Source: CAD feature listing. Evaluate the final solid. Frame: model axes, mm. A direction names the side the tool comes from. Coordinates: 2 decimals unless noted, no trailing zeros. Write each loop counter-clockwise with the first axis right and the second up, starting at its lowest first coordinate (ties: lowest second). Pieces come first, ordered by that corner, then holes. Notation, with made-up numbers: M 57.25,2 L 106.25,2 A21 cw 106.25,12 Z; hole C 86,73 d2. An arc over 180 degrees is marked long. Answer as CSV lines item,"result". Start each with the question number.
1. Section C-C on z = -18. Return the cut outline in (x, y) (3 decimals).
2. Reachability of faces 4 (the face through (-47, 6.35, 0)), 5 (the face through (-7.7, 4.7, -10.1)) from +Z, -Z, +X, -X, +Y, -Y: full face, straight path, thin tool, end or side. Return the list, or none.
3. Section B-B on x = -9.5. Return the cut outline in (y, z) (3 decimals), plus the area to 3 significant figures.
4. Mould query, pull axis Z, two halves, no side actions, for faces 1 (the face through (-63.85, 1.57, -14.18)), 2 (the face through (0.109, 3.47, -3.046)), 3 (the face through (0, 6.35, 47)). Classes: pulls with the +Z half, pulls with the -Z half, needs draft (parallel to the pull), parting line crosses it, or undercut.
5. Section A-A on y = 2. Return the cut outline in (x, z) (3 decimals).
6. Line query: probe 1 along X at (y, z) = (3.55, 0); probe 2 along Y at (x, z) = (-44, -34) (3 decimals); probe 3 along X at (y, z) = (2.75, 1). Output: solid intervals per line, ascending. Write a range as [from, to].
7. Contact query for flat-ended pins moving along their axis: pin 1 Ø3.5 at (x, z) = (0, 0) entering from +Y; pin 2 Ø1.5 at (y, z) = (1.5, 8.5) entering from +X; pin 3 Ø12 at (x, z) = (-26, 24) entering from +Y (3 decimals); pin 4 Ø3 at (y, z) = (5, 29) entering from -X. Output: stop coordinate, or through.
8. Section D-D on x = 15. Return the cut outline in (y, z) (3 decimals), plus the area to 3 significant figures.
```python
from build123d import *

# Parameters (mm, degrees)
SKETCH1_R           = 65.405
BOSS_EXTRUDE1_DEPTH = 3.175
SKETCH2_R           = 12.7
BOSS_EXTRUDE2_DEPTH = 3.175
CUT_EXTRUDE1_DEPTH  = 5.842
SKETCH4_R           = 7.032250482
BOSS_EXTRUDE3_DEPTH = 3.175
FILLET3_R           = 6.35


with BuildPart() as part:
    # Sketch1 → Boss-Extrude1 (new body)
    with BuildSketch(Plane(origin=(0, 0, 0), x_dir=(1, 0, 0), z_dir=(0, 1, 0))):
        with Locations(Location((0, 0, 0), (0, 0, 270))):
            Circle(SKETCH1_R)
    extrude(amount=BOSS_EXTRUDE1_DEPTH)

    # Sketch2 → Boss-Extrude2 (add)
    with BuildSketch(Plane(origin=(0, 3.175, 0), x_dir=(1, 0, 0), z_dir=(0, 1, 0))):
        with Locations(Location((0, 0, 0), (0, 0, 270))):
            Circle(SKETCH2_R)
    extrude(amount=BOSS_EXTRUDE2_DEPTH)

    # Sketch3 → Cut-Extrude1 (cut)
    with BuildSketch(Plane(origin=(0, 6.35, 0), x_dir=(1, 0, 0), z_dir=(0, 1, 0))):
        with BuildLine():
            Line((-1.684845394, -2.54), (1.684845394, -2.54))
            ThreePointArc((1.684845394, -2.54), (0, 3.048), (-1.684845394, -2.54))
        make_face()
    extrude(amount=-CUT_EXTRUDE1_DEPTH, mode=Mode.SUBTRACT)

    # Sketch4 → Boss-Extrude3 (add)
    with BuildSketch(Plane(origin=(0, 3.175, 0), x_dir=(1, 0, 0), z_dir=(0, 1, 0))):
        with Locations(Location((0, 46.973149897, 0), (0, 0, 270))):
            Circle(SKETCH4_R)
        with Locations(Location((46.973149897, 0, 0), (0, 0, 270))):
            Circle(SKETCH4_R)
        with Locations(Location((0, -46.973149897, 0), (0, 0, 270))):
            Circle(SKETCH4_R)
        with Locations(Location((-46.973149897, 0, 0), (0, 0, 270))):
            Circle(SKETCH4_R)
    extrude(amount=BOSS_EXTRUDE3_DEPTH)

    # Fillet3
    # the kernel refuses this fillet: 6.35 mm, written as the material it takes off along each edge
    with BuildSketch(Plane(origin=(0, 6.35, -46.973149897), x_dir=(0, 0, 1), z_dir=(-1, 0, 0))) as fillet3_piece_1:
        with BuildLine():
            CenterArc((1.532989168, -6.35), FILLET3_R, 30, 60)
            Line((1.532989168, 0), (1.532989168, 0.127))
            Line((1.532989168, 0.127), (7.032250482, 0.127))
            Line((7.032250482, 0.127), (7.159250482, 0))
            ThreePointArc((7.159250482, 0), (7.159250482, -1.5875), (7.142235708, -3.1115))
            Line((7.142235708, -3.1115), (7.032250482, -3.175))
        make_face()
    revolve(axis=Axis((0, 6.35, -46.973149897), (0, 1, 0)), mode=Mode.SUBTRACT)
    with BuildSketch(Plane(origin=(46.973149897, 6.35, 0), x_dir=(0, 0, 1), z_dir=(-1, 0, 0))) as fillet3_piece_2:
        with BuildLine():
            CenterArc((1.532989168, -6.35), FILLET3_R, 30, 60)
            Line((1.532989168, 0), (1.532989168, 0.127))
            Line((1.532989168, 0.127), (7.032250482, 0.127))
            Line((7.032250482, 0.127), (7.159250482, 0))
            ThreePointArc((7.159250482, 0), (7.159250482, -1.5875), (7.142235708, -3.1115))
            Line((7.142235708, -3.1115), (7.032250482, -3.175))
        make_face()
    revolve(axis=Axis((46.973149897, 6.35, 0), (0, 1, 0)), mode=Mode.SUBTRACT)
    with BuildSketch(Plane(origin=(0, 6.35, 46.973149897), x_dir=(0, 0, 1), z_dir=(-1, 0, 0))) as fillet3_piece_3:
        with BuildLine():
            CenterArc((1.532989168, -6.35), FILLET3_R, 30, 60)
            Line((1.532989168, 0), (1.532989168, 0.127))
            Line((1.532989168, 0.127), (7.032250482, 0.127))
            Line((7.032250482, 0.127), (7.159250482, 0))
            ThreePointArc((7.159250482, 0), (7.159250482, -1.5875), (7.142235708, -3.1115))
            Line((7.142235708, -3.1115), (7.032250482, -3.175))
        make_face()
    revolve(axis=Axis((0, 6.35, 46.973149897), (0, 1, 0)), mode=Mode.SUBTRACT)
    with BuildSketch(Plane(origin=(-46.973149897, 6.35, 0), x_dir=(0, 0, 1), z_dir=(-1, 0, 0))) as fillet3_piece_4:
        with BuildLine():
            CenterArc((1.532989168, -6.35), FILLET3_R, 30, 60)
            Line((1.532989168, 0), (1.532989168, 0.127))
            Line((1.532989168, 0.127), (7.032250482, 0.127))
            Line((7.032250482, 0.127), (7.159250482, 0))
            ThreePointArc((7.159250482, 0), (7.159250482, -1.5875), (7.142235708, -3.1115))
            Line((7.142235708, -3.1115), (7.032250482, -3.175))
        make_face()
    revolve(axis=Axis((-46.973149897, 6.35, 0), (0, 1, 0)), mode=Mode.SUBTRACT)


solid = part.part
```
Values:
1,outline,"M -62.879,0 L 62.879,0 L 62.879,3.175 L -62.879,3.175 Z"
2,face 4,"+Z, -Z, +X, -X, +Y"
2,face 5,"+Y"
3,outline,"M 0,-64.711 L 3.175,-64.711 L 3.175,-8.429 L 6.35,-8.429 L 6.35,8.429 L 3.175,8.429 L 3.175,64.711 L 0,64.711 Z"
3,area,"464 mm²"
4,face 1,"parting line crosses it"
4,face 2,"undercut"
4,face 3,"needs draft"
5,outline,"C 0,0 d130.81; hole M -1.685,2.54 A3.048 ccw long 1.685,2.54 Z"
6,probe 1,"[-53.77, -40.18], [-12.7, -3.05], [3.05, 12.7], [40.18, 53.77]"
6,probe 2,"[0, 3.175]"
6,probe 3,"[-65.4, -2.88], [2.88, 65.4]"
7,pin 1,"y = 0.51"
7,pin 2,"x = 64.94"
7,pin 3,"y = 3.175"
7,pin 4,"through"
8,outline,"M 0,-63.662 L 3.175,-63.662 L 3.175,63.662 L 0,63.662 Z"
8,area,"404 mm²"
